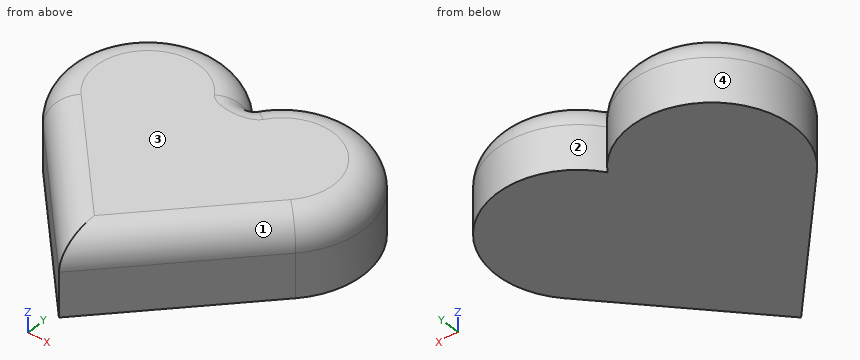
from build123d import *

# Parameters (mm, degrees)
PAD_DEPTH = 2.5
FILLET_R  = 1


with BuildPart() as part:
    # Sketch → Pad (new body)
    with BuildSketch(Plane.XY):
        with BuildLine():
            ThreePointArc((0, 0), (-3.989817, 0.583782), (-4.272701, -3.438583))
            Line((-4.272701, -3.438583), (0, -8))
            Line((4.272701, -3.438583), (0, -8))
            ThreePointArc((4.272701, -3.438583), (3.989817, 0.583782), (0, 0))
        make_face()
    extrude(amount=PAD_DEPTH)

    # Fillet
    fillet_edges = [part.edges().sort_by_distance(p)[0] for p in [
        (-3.989817, 0.583782, 2.5),
        (-2.13635, -5.719291, 2.5),
        (2.13635, -5.719291, 2.5),
        (3.989817, 0.583782, 2.5),
    ]]
    fillet(fillet_edges, radius=FILLET_R)


solid = part.part
Check sheet for the modelled part. Datum: model origin and axes. Units: mm. Face numbers are marked on the shaded views. Give positions to 0.01 mm unless a question says otherwise; leave off trailing zeros. Write each loop counter-clockwise with the first axis right and the second up, starting at its lowest first coordinate (ties: lowest second). Pieces come first, ordered by that corner, then holes. Notation, with made-up numbers: (-21.75, 80.5) -> (-11.75, 80.5) arc R19 ccw to (-11.75, 115.5) -> close; hole circle Ø6 at (48, 50). An arc over 180 degrees is marked (long way). Use one line per item in the form item = value. Start each with the question number.
1. Go/stop test with flat-tipped pins: P1, Ø1.5, axis at y = -5.5, z = 1, coming from the +X side; P2, Ø1.5, axis at y = -0.5, z = 0.5, coming from the +X side. Record where each tip stops, or that it passes through.
2. Mould release check, pull along X, two halves, no side actions. Record for the marked faces 1, 2, 3 and 4: pulls with the +X half, pulls with the -X half, needs draft (parallel to the pull), parting line crosses it, or undercut.
3. Thickness scan on line 1 along X through (y, z) = (-6.5, 0.2); line 2 along Z through (x, y) = (-3, 0.25); line 3 along X through (y, z) = (-2.75, 1.25). Record the ranges inside material, lowest first. Write a range as from..to.
4. Section check A-A (z = 0.4). Record the cut outline in (x, y).
Conclusion:
q1.P1 = 3.04
q1.P2 = 5
q2.face_1 = pulls with the +X half
q2.face_2 = undercut
q2.face_3 = needs draft
q2.face_4 = undercut
q3.line_1 = -1.41..1.41
q3.line_2 = 0..2.48
q3.line_3 = -4.74..4.74
q4.outline = (-4.27, -3.44) -> (0, -8) -> (4.27, -3.44) arc R2.75 ccw (long way) to (0, 0) arc R2.75 ccw (long way) to start
